Job drawing, mm, ordinate dimensions from the low corner. One solid piece. A direction names the side the tool comes from. Round coordinates to 2 decimals unless told otherwise and drop trailing zeros. Loops run counter-clockwise (first coordinate to the right, second up) from the corner with the lowest first, then second, coordinate; pieces in that order, holes last. Notation, with made-up numbers: M -3.5,-20 L 17.5,-20 A18 ccw 17.5,-7 Z; hole C 22.25,82 d1. An arc over 180 degrees is marked long. Put each result on its own line as item: value. Start each with the question number.
1) Slice it at D-D on z = 58. Give the cut face in (x, y).
2) Slice it at C-C on z = 19. Give the cut face in (x, y) (1 decimal).
3) Which spindle directions (+Z, -Z, +X, -X, +Y, -Y) get a long thin tool onto all of the face, cutting with end or side? Do the marked faces 1, 2 and 3. Say none if no direction does.
4) Pull direction Y, two halves, no side cores. Call the marked faces 4, 5 and 6: +Y half, -Y half, draft (parallel to the pull), parting line (faces both ways), or undercut.
5) Slice it at B-B on x = 33.5. Give the cut face in (y, z) (1 decimal), then the cut area to 3 significant figures.
6) Probe line 1 along X through (y, z) = (12, 20); line 2 along X through (y, z) = (29, 59); line 3 along Z through (x, y) = (5, 42.5). List the from-to ranges inside material, lowest first.
7) Slice it at A-A on y = 35. Give the cut face in (x, z) (1 decimal).
8) Drop flat-ended pins along their axis: pin 1 Ø2 at (x, z) = (32.5, 49) entering from -Y; pin 2 Ø10 at (x, y) = (61, 18.5) entering from +Z; pin 3 Ø6.5 at (x, y) = (45.5, 43.5) entering from -Z. Give the stop position or say it passes through.
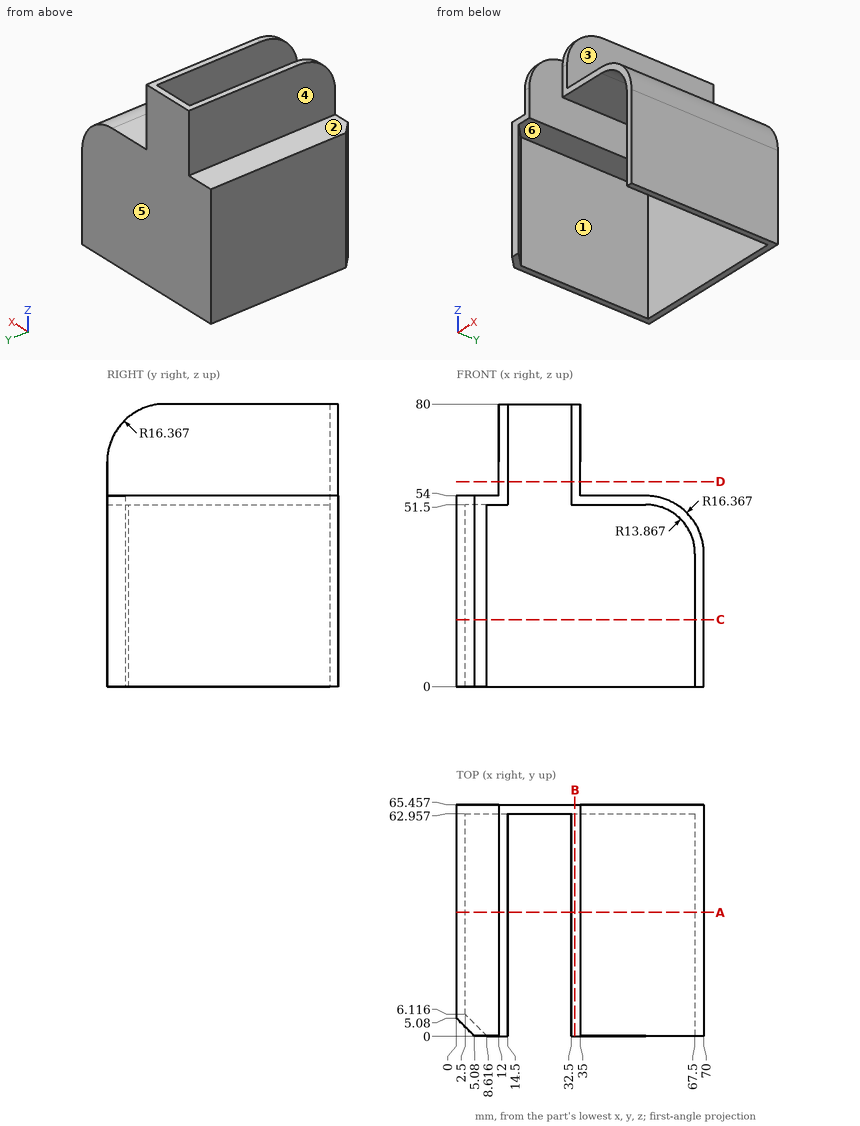
Recorded:
1. outline: M 12,0 L 14.5,0 L 14.5,62.96 L 32.5,62.96 L 32.5,0 L 35,0 L 35,65.46 L 12,65.46 Z
2. outline: M 0,5.1 L 5.1,0 L 8.6,0 L 2.5,6.1 L 2.5,63 L 67.5,63 L 67.5,0 L 70,0 L 70,65.5 L 0,65.5 Z
3. face 1: -Z
3. face 2: +Z, -X, +Y, -Y
3. face 3: +Z, +X, +Y, -Y
4. face 4: draft
4. face 5: +Y half
4. face 6: undercut
5. outline: M 0,51.5 L 63,51.5 L 63,0 L 65.5,0 L 65.5,80 L 16.4,80 A16.4 ccw 0,63.6 Z
5. area: 1,940 mm2
6. line 1: x = 0 to 2.5, 67.5 to 70
6. line 2: x = 12 to 14.5, 32.5 to 35
6. line 3: z = 51.5 to 54
7. outline: M 0,0 L 2.5,0 L 2.5,51.5 L 14.5,51.5 L 14.5,80 L 12,80 L 12,54 L 0,54 Z; M 32.5,51.5 L 53.6,51.5 A13.9 cw 67.5,37.6 L 67.5,0 L 70,0 L 70,37.6 A16.4 ccw 53.6,54 L 35,54 L 35,80 L 32.5,80 Z
8. pin 1: stops at y = 62.96
8. pin 2: stops at z = 53.83
8. pin 3: stops at z = 51.5
